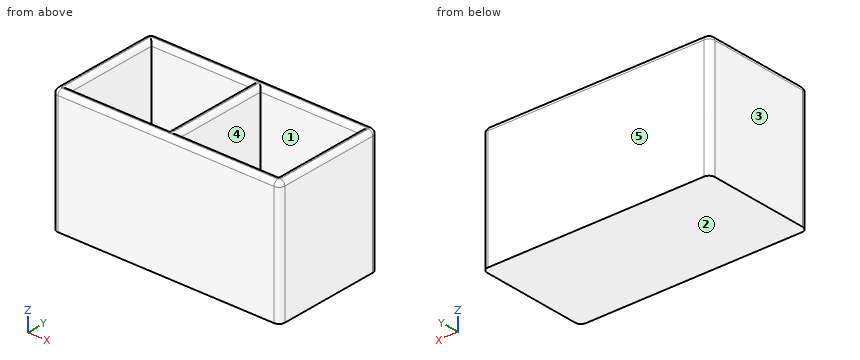
from build123d import *

# Parameters (mm, degrees)
F0_W         = 152.4
F0_H         = 76.2
F1_DEPTH     = 6.35
F2_W         = 152.4
F2_H         = 76.2
F2_W_2       = 66.675
F2_H_2       = 63.5
F3_DEPTH     = 76.2
F4_R         = 3.048
F5_T1_DEPTH  = 92.329
F5_T4_ANGLE  = 90
F5_T6_ANGLE  = 90
F5_T8_ANGLE  = 90
F5_T10_ANGLE = 90


# Not quite as in the source:
# - a fillet or chamfer that OpenCascade refuses, or shapes differently, is made with other operations: its cross-section is extruded or revolved along the edge and cut away or added
# - a feature names something its author has since deleted; it is built from what else it names


with BuildPart() as f1:
    # F0 (on Top) → F1 (new body)
    with BuildSketch(Plane.XY):
        with Locations((-119.875261867, -15.1447099686)):
            Rectangle(F0_W, F0_H)
    extrude(amount=F1_DEPTH)

    # F2 (on face) → F3 (join)
    with BuildSketch(Plane.XY.offset(6.35)):
        with Locations((-119.875261867, -15.1447099686)):
            Rectangle(F2_W, F2_H)
        with Locations((-156.387761867, -15.1447099686)):
            Rectangle(F2_W_2, F2_H_2, mode=Mode.SUBTRACT)
        with Locations((-83.362761867, -15.1447099686)):
            Rectangle(F2_W_2, F2_H_2, mode=Mode.SUBTRACT)
    extrude(amount=F3_DEPTH)

    # F4
    f4_edges = [f1.edges().sort_by_distance(p)[0] for p in [
        (-196.075262, -15.14471, 82.55),
        (-119.875262, 22.95529, 82.55),
        (-43.675262, -15.14471, 82.55),
        (-119.875262, -53.24471, 82.55),
        (-123.050262, -15.14471, 82.55),
        (-156.387762, -46.89471, 82.55),
        (-189.725262, -15.14471, 82.55),
        (-156.387762, 16.60529, 82.55),
        (-83.362762, 16.60529, 82.55),
        (-50.025262, -15.14471, 82.55),
        (-83.362762, -46.89471, 82.55),
        (-116.700262, -15.14471, 82.55),
    ]]
    fillet(f4_edges, radius=F4_R)

    # F5: fillet of radius 3.9116 on 4 edges, made by hand

    # F5_s2 → F5_t1 (cut)
    with BuildSketch(Plane.XY.offset(-9.779)):
        with BuildLine():
            ThreePointArc((-47.586861867, -53.2447099686), (-44.8209429818, -52.0990288539), (-43.675261867, -49.3331099686))
            Line((-43.675261867, -49.3331099686), (-43.675261867, -53.2447099686))
            Line((-43.675261867, -53.2447099686), (-47.586861867, -53.2447099686))
        make_face()
        with BuildLine():
            ThreePointArc((-43.675261867, 19.0436900314), (-44.8209429818, 21.8096089167), (-47.586861867, 22.9552900314))
            Line((-47.586861867, 22.9552900314), (-43.675261867, 22.9552900314))
            Line((-43.675261867, 22.9552900314), (-43.675261867, 19.0436900314))
        make_face()
        with BuildLine():
            ThreePointArc((-192.163661867, -53.2447099686), (-194.9295807523, -52.0990288539), (-196.075261867, -49.3331099686))
            Line((-196.075261867, -49.3331099686), (-196.075261867, -53.2447099686))
            Line((-196.075261867, -53.2447099686), (-192.163661867, -53.2447099686))
        make_face()
        with BuildLine():
            ThreePointArc((-196.075261867, 19.0436900314), (-194.9295807523, 21.8096089167), (-192.163661867, 22.9552900314))
            Line((-192.163661867, 22.9552900314), (-196.075261867, 22.9552900314))
            Line((-196.075261867, 22.9552900314), (-196.075261867, 19.0436900314))
        make_face()
    extrude(amount=F5_T1_DEPTH, mode=Mode.SUBTRACT)

    # F5_s3 → F5_t4 (revolve, cut)
    with BuildSketch(Plane.YZ.offset(-192.163661867)):
        with BuildLine():
            ThreePointArc((19.9072900314, 82.55), (22.0625515005, 81.6572614691), (22.9552900314, 79.502))
            Line((22.9552900314, 79.502), (22.9552900314, 82.55))
            Line((22.9552900314, 82.55), (19.9072900314, 82.55))
        make_face()
    revolve(axis=Axis((-192.163661867, 19.0436900314, 82.55), (0, 0, 1)), revolution_arc=F5_T4_ANGLE, mode=Mode.SUBTRACT)

    # F5_s5 → F5_t6 (revolve, cut)
    with BuildSketch(Plane.XZ.offset(49.3331099686)):
        with BuildLine():
            ThreePointArc((-193.027261867, 82.55), (-195.1825233361, 81.6572614691), (-196.075261867, 79.502))
            Line((-196.075261867, 79.502), (-196.075261867, 82.55))
            Line((-196.075261867, 82.55), (-193.027261867, 82.55))
        make_face()
    revolve(axis=Axis((-192.163661867, -49.3331099686, 82.55), (0, 0, 1)), revolution_arc=F5_T6_ANGLE, mode=Mode.SUBTRACT)

    # F5_s7 → F5_t8 (revolve, cut)
    with BuildSketch(Plane.XZ.offset(-19.0436900314)):
        with BuildLine():
            ThreePointArc((-46.723261867, 82.55), (-44.568000398, 81.6572614691), (-43.675261867, 79.502))
            Line((-43.675261867, 79.502), (-43.675261867, 82.55))
            Line((-43.675261867, 82.55), (-46.723261867, 82.55))
        make_face()
    revolve(axis=Axis((-47.586861867, 19.0436900314, 82.55), (0, 0, 1)), revolution_arc=F5_T8_ANGLE, mode=Mode.SUBTRACT)

    # F5_s9 → F5_t10 (revolve, cut)
    with BuildSketch(Plane.YZ.offset(-47.586861867)):
        with BuildLine():
            ThreePointArc((-50.1967099686, 82.55), (-52.3519714376, 81.6572614691), (-53.2447099686, 79.502))
            Line((-53.2447099686, 79.502), (-53.2447099686, 82.55))
            Line((-53.2447099686, 82.55), (-50.1967099686, 82.55))
        make_face()
    revolve(axis=Axis((-47.586861867, -49.3331099686, 82.55), (0, 0, 1)), revolution_arc=F5_T10_ANGLE, mode=Mode.SUBTRACT)


solid = f1.part
Can you work these out from the model? Positions are in its coordinate system, mm. Face numbers are marked on the shaded views. A direction names the side the tool comes from. Round coordinates to 2 decimals unless told otherwise and drop trailing zeros. Write each loop counter-clockwise with the first axis right and the second up, starting at its lowest first coordinate (ties: lowest second). Pieces come first, ordered by that corner, then holes. Notation, with made-up numbers: M -30.5,5 L 4.5,5 A13 ccw 4.5,11 Z; hole C 15.25,82.5 d5. An arc over 180 degrees is marked long. Use a Markdown table: item, result.
Item 1: If I drill on line 1 along X through (y, z) = (-5, 15); line 2 along Y through (x, z) = (-71, 19.5); line 3 along Z through (x, y) = (-140, -42.5), over which ranges is the centre line in solid material (lowest first)? Write a range as [from, to].
Found:
| item | result |
|---|---|
| line 1 | x = [-196.08, -189.73], [-123.05, -116.7], [-50.03, -43.68] |
| line 2 | y = [-53.24, -46.89], [16.61, 22.96] |
| line 3 | z = [0, 6.35] |
Item 2: We'd pull the mould along Y, two halves only. Please class the marked faces 3, 4 and 5: released by +Y, released by -Y, zero draft, split by the parting line, or undercut.
Found:
| item | result |
|---|---|
| face 3 | zero draft |
| face 4 | undercut |
| face 5 | released by +Y |
Item 3: I want a section at A-A (z = 77.5). List the corners of the cut face in (x, y) for me.
Found:
| item | result |
|---|---|
| outline | M -196.08,-49.33 A3.91 ccw -192.16,-53.24 L -47.59,-53.24 A3.91 ccw -43.68,-49.33 L -43.68,19.04 A3.91 ccw -47.59,22.96 L -192.16,22.96 A3.91 ccw -196.08,19.04 Z; hole M -189.73,-46.89 L -123.05,-46.89 L -123.05,16.61 L -189.73,16.61 Z; hole M -116.7,-46.89 L -50.03,-46.89 L -50.03,16.61 L -116.7,16.61 Z |
Item 4: Which directions (+Z, -Z, +X, -X, +Y, -Y) give clear straight access to the entire face, cutting with the end or side of a thin tool? Please do the marked faces 1 and 2.
Found:
| item | result |
|---|---|
| face 1 | +Z |
| face 2 | -Z, +X, -X, +Y, -Y |
Item 5: I want a section at B-B (y = -25). List the corners of the cut face in (x, z) for me, and give its area (3 significant figures).
Found:
| item | result |
|---|---|
| outline | M -196.08,0 L -43.68,0 L -43.68,79.5 A3.05 ccw -46.72,82.55 L -46.98,82.55 A3.05 ccw -50.03,79.5 L -50.03,6.35 L -116.7,6.35 L -116.7,79.5 A3.05 ccw -119.75,82.55 L -120,82.55 A3.05 ccw -123.05,79.5 L -123.05,6.35 L -189.73,6.35 L -189.73,79.5 A3.05 ccw -192.77,82.55 L -193.03,82.55 A3.05 ccw -196.08,79.5 Z |
| area | 2,410 mm2 |
Item 6: I want a section at C-C (x = -77). List the corners of the cut face in (y, z) for me, and give its area (3 significant figures).
Found:
| item | result |
|---|---|
| outline | M -53.24,0 L 22.96,0 L 22.96,79.5 A3.05 ccw 19.91,82.55 L 19.65,82.55 A3.05 ccw 16.61,79.5 L 16.61,6.35 L -46.89,6.35 L -46.89,79.5 A3.05 ccw -49.94,82.55 L -50.2,82.55 A3.05 ccw -53.24,79.5 Z |
| area | 1,440 mm2 |
Item 7: For pin 1 Ø19 at (x, y) = (-147, -2.5) entering from +Z, with a flat end and sliding along its axis, tell me the tip position at first contact or that it passes through.
Found:
| item | result |
|---|---|
| pin 1 | stops at z = 6.35 |
